Autodesk Inventor part; units mm, degrees
ref_plane "YZ Plane" through (0, 0, 0) normal (1, 0, 0) x (0, 1, 0)
ref_plane "XZ Plane" through (0, 0, 0) normal (0, 1, 0) x (-1, 0, 0)
ref_plane "XY Plane" through (0, 0, 0) normal (0, 0, 1) x (1, 0, 0)
sketch "Sketch1" plane through (0.0001, 0, 0) normal (0, 0, 1) x (1, 0, 0)
  line L0 (47.5003, -5) -> (47.5003, 4.9999)
  line L1 (47.5003, 4.9999) -> (42.5003, 4.9999)
  line L2 (42.5003, 4.9999) -> (42.5003, 9.9999)
  line L3 (42.5003, 9.9999) -> (22.4998, 10)
  line L4 (22.4998, 10) -> (22.4998, 5)
  line L5 (22.4998, 5) -> (-22.5002, 5)
  line L6 (-22.5002, 5) -> (-22.5002, 10)
  line L7 (-22.5002, 10) -> (-42.5005, 10)
  line L8 (-42.5005, 10) -> (-42.5003, 5)
  line L9 (-42.5003, 5) -> (-47.5003, 4.9999)
  line L10 (-47.5003, 4.9999) -> (-47.5, -5)
  line L11 (-47.5, -5) -> (-42.5, -4.9999)
  line L12 (-42.5, -4.9999) -> (-42.4999, -10)
  line L13 (-42.4999, -10) -> (42.5003, -10)
  line L14 (42.5003, -10) -> (42.5003, -5)
  line L15 (42.5003, -5) -> (47.5003, -5)
  circle A0 centre (-30, 0) radius 2
  circle A1 centre (30, 0) radius 2
  point P0 (-0.0005, 0)
extrude "AP" add sketch "Sketch1" along normal blind 5
properties part number "AP"
Design review of the part built by this model. Coordinates are the model's own, in mm. A direction names the side the tool comes from. Give positions to 0.01 mm unless a question says otherwise; leave off trailing zeros. Order: outer loops, then holes, each group sorted by start corner. A loop starts at its lowest first (then second) coordinate and runs counter-clockwise, first axis right, second up. Notation, with made-up numbers: (37.5, 25.5) - (65.5, 25.5) arc R11 cw to (65.5, 37.5) - close; hole circle Ø5 at (8, -23). An arc over 180 degrees is marked (long way). Write item = value, one per line. Start each with the question number.
Q1. Clearance check with flat-ended pins moving along their axes: pin 1 Ø2.5 at (x, z) = (44.5, 3.5) entering from -Y; pin 2 Ø1.5 at (x, z) = (-44.5, 3.5) entering from +Y; pin 3 Ø1.5 at (y, z) = (-7.5, 2.5) entering from -X. State where each tip first meets the part, or that it passes through.
Q2. To check wall thickness, follow L1, parallel to X at y = 6.5, z = 1.6; L2, parallel to X at y = -5.5, z = 4.2; L3, parallel to Y at x = -9, z = 0.3. State the ranges of each line that lie inside material, in increasing order. Write a range as from..to.
Q3. We need section A-A on y = 8.5. State the section outline as (x, z) points.
Q4. We need section C-C on y = 0. State the section outline as (x, z) points.
Q5. We need section D-D on x = -2.5. State the section outline as (y, z) points, plus the area to 3 significant figures.
Q6. We need section B-B on z = 2. State the section outline as (x, y) points, plus the area to 3 significant figures.
Q7. Tool access review of faces 1 (the face through (42.5, 7, 2)), 2 (the face through (22.5, 8, 2)), 3 (the face through (45, -5, 2)): name each direction out of +Z, -Z, +X, -X, +Y, -Y from which nothing blocks a thin tool from reaching the whole face with its end or side.
Q8. Mouldability with a two-part tool opening along Y and no side actions: class faces 4 (the face through (28, 0, 2)), 5 (the face through (47.5, 0, 2)), 6 (the face through (0, 5, 2)) as released by +Y, released by -Y, zero draft, split by the parting line, or undercut.
Working result:
q1.pin_1 = -5
q1.pin_2 = 5
q1.pin_3 = -42.5
q2.L1 = -42.5..-22.5, 22.5..42.5
q2.L2 = -42.5..42.5
q2.L3 = -10..5
q3.outline = (-42.5, 0) - (-22.5, 0) - (-22.5, 5) - (-42.5, 5) - close; (22.5, 0) - (42.5, 0) - (42.5, 5) - (22.5, 5) - close
q4.outline = (-47.5, 0) - (-32, 0) - (-32, 5) - (-47.5, 5) - close; (-28, 0) - (28, 0) - (28, 5) - (-28, 5) - close; (32, 0) - (47.5, 0) - (47.5, 5) - (32, 5) - close
q5.outline = (-10, 0) - (5, 0) - (5, 5) - (-10, 5) - close
q5.area = 75.0 mm²
q6.outline = (-47.5, -5) - (-42.5, -5) - (-42.5, -10) - (42.5, -10) - (42.5, -5) - (47.5, -5) - (47.5, 5) - (42.5, 5) - (42.5, 10) - (22.5, 10) - (22.5, 5) - (-22.5, 5) - (-22.5, 10) - (-42.5, 10) - (-42.5, 5) - (-47.5, 5) - close; hole circle Ø4 at (-30, 0); hole circle Ø4 at (30, 0)
q6.area = 1,550 mm²
q7.face_1 = +Z, -Z, +X, +Y
q7.face_2 = +Z, -Z, +Y
q7.face_3 = +Z, -Z, +X, -Y
q8.face_4 = undercut
q8.face_5 = zero draft
q8.face_6 = released by +Y
